```python
from build123d import *

# Parameters (mm, degrees)
BOSS_EXTRUDE1_DEPTH      = 35
SKETCH2_W                = 11
SKETCH2_H                = 21
BOSS_EXTRUDE3_DEPTH      = 150
BOSS_EXTRUDE4_DEPTH      = 35
SKETCH4_W                = 16
SKETCH4_H                = 14
BOSS_EXTRUDE5_DEPTH      = 150
SKETCH5_W                = 14
SKETCH5_H                = 14
BOSS_EXTRUDE6_DEPTH      = 25
SKETCH6_W                = 121
SKETCH6_H                = 207.00216397
BOSS_EXTRUDE7_DEPTH      = 5
SKETCH7_R                = 11
BOSS_EXTRUDE8_DEPTH      = 10
BOSS_EXTRUDE8_DEPTH_BACK = 230
SKETCH8_W                = 46
SKETCH8_H                = 122
CUT_EXTRUDE1_DEPTH       = 5


with BuildPart() as part:
    # Sketch1 → Boss-Extrude1 (new body)
    with BuildSketch(Plane.XY):
        with BuildLine():
            Line((0, 0), (150, 0))
            ThreePointArc((150, 0), (79.056941504, 37.170824513), (0, 50))
            Line((0, 50), (0, 0))
        make_face()
    extrude(amount=BOSS_EXTRUDE1_DEPTH)

    # Sketch2 → Boss-Extrude3 (add)
    with BuildSketch(Plane.XY.offset(35)):
        with Locations((9.5, 24.924601572)):
            Rectangle(SKETCH2_W, SKETCH2_H)
    extrude(amount=BOSS_EXTRUDE3_DEPTH)

    # Sketch3 → Boss-Extrude4 (add)
    with BuildSketch(Plane.XY.offset(185)):
        with BuildLine():
            Line((150, 0), (0, 0))
            Line((0, 0), (0, 50))
            ThreePointArc((0, 50), (79.056941504, 37.170824513), (150, 0))
        make_face()
    extrude(amount=BOSS_EXTRUDE4_DEPTH)

    # Sketch4 → Boss-Extrude5 (add)
    with BuildSketch(Plane(origin=(0, 0, 185), x_dir=(-1, 0, 0), z_dir=(0, 0, -1))):
        with Locations((-102, 13)):
            Rectangle(SKETCH4_W, SKETCH4_H)
    extrude(amount=BOSS_EXTRUDE5_DEPTH)

    # Sketch5 → Boss-Extrude6 (add)
    with BuildSketch(Plane.XZ):
        with Locations((23, 202.48216397)):
            Rectangle(SKETCH5_W, SKETCH5_H)
        with Locations((23, 17.48)):
            Rectangle(SKETCH5_W, SKETCH5_H)
        with Locations((122, 202.48216397)):
            Rectangle(SKETCH5_W, SKETCH5_H)
        with Locations((122, 17.48)):
            Rectangle(SKETCH5_W, SKETCH5_H)
    extrude(amount=BOSS_EXTRUDE6_DEPTH)

    # Sketch6 → Boss-Extrude7 (add)
    with BuildSketch(Plane(origin=(0, -25, 0), x_dir=(-1, 0, 0), z_dir=(0, -1, 0))):
        with Locations((-72.5, -109.981081985)):
            Rectangle(SKETCH6_W, SKETCH6_H)
    extrude(amount=BOSS_EXTRUDE7_DEPTH)

    # Sketch7 → Boss-Extrude8 (add, two sides)
    with BuildSketch(Plane(origin=(0, 0, 0), x_dir=(-1, 0, 0), z_dir=(0, 0, -1))) as boss_extrude8_sk:
        with Locations((-63, 18)):
            Circle(SKETCH7_R)
    extrude(amount=BOSS_EXTRUDE8_DEPTH)
    extrude(boss_extrude8_sk.sketch, amount=-BOSS_EXTRUDE8_DEPTH_BACK)

    # Sketch8 → Cut-Extrude1 (cut)
    with BuildSketch(Plane.XZ.offset(30)):
        with Locations((65, 109.98216397)):
            Rectangle(SKETCH8_W, SKETCH8_H)
    extrude(amount=-CUT_EXTRUDE1_DEPTH, mode=Mode.SUBTRACT)


solid = part.part
```
Geometry check sheet. Reference: the model listing, model coordinates, mm. A direction names the side the tool comes from. Give positions to 0.01 mm unless a question says otherwise; leave off trailing zeros. Order: outer loops, then holes, each group sorted by start corner. A loop starts at its lowest first (then second) coordinate and runs counter-clockwise, first axis right, second up.
1. Section check B-B, the plane z = 121.5. Enter the section's corners in (x, y).
2. Gauge pin test, flat ends, axial feed: pin 1 Ø6.5 at (y, z) = (26.5, 145.5) entering from -X; pin 2 Ø5.5 at (y, z) = (-28, 97.5) entering from -X; pin 3 Ø1.5 at (y, z) = (-26.5, 82.5) entering from +X. Record the tip position at first contact, or that the pin passes through.
3. Release check for a two-part mould opening along X. For faces 1 (the face through (9, 14.425, 109)), 2 (the face through (80.124, 36.812, 17.255)), 3 (the face through (88, -28, 109)), 4 (the face through (12, -27, 111)) record: pulls with the +X half, pulls with the -X half, needs draft (parallel to the pull), parting line crosses it, or undercut.
4. Section check D-D, the plane x = 63. Enter the section's corners in (y, z).
5. Access from +Z, -Z, +X, -X, +Y, -Y to the whole of each face (thin tool, end or side, straight path). Record for faces 5 (the face through (102, 20, 111)), 6 (the face through (15, 25, 109)), 7 (the face through (115, -12, 17)), 8 (the face through (65, -28, 48.982)), 9 (the face through (71.73, 11.31, -4.93)).
6. Section check A-A, the plane z = 31.5. Enter the section's corners in (x, y), and give its area (3 significant figures).
7. Thickness scan on L1, parallel to Y at x = 104.5, z = 98; L2, parallel to Z at x = 58.5, y = 6.5; L3, parallel to Z at x = 120, y = -24.5. Record the ranges inside material, lowest first.
8. Section check C-C, the plane x = 97.5. Enter the section's corners in (y, z), and give its area (3 significant figures).
Values follow:
1. outline: (4, 14.42) - (15, 14.42) - (15, 35.42) - (4, 35.42) - close; (12, -30) - (42, -30) - (42, -25) - (12, -25) - close; circle Ø22 at (63, 18); (88, -30) - (133, -30) - (133, -25) - (88, -25) - close; (94, 6) - (110, 6) - (110, 20) - (94, 20) - close
2. pin 1: stops at x = 4
2. pin 2: stops at x = 12
2. pin 3: stops at x = 133
3. face 1: needs draft
3. face 2: pulls with the +X half
3. face 3: undercut
3. face 4: pulls with the -X half
4. outline: (-30, 6.48) - (-25, 6.48) - (-25, 48.98) - (-30, 48.98) - close; (-30, 170.98) - (-25, 170.98) - (-25, 213.48) - (-30, 213.48) - close; (0, 0) - (7, 0) - (7, -10) - (29, -10) - (29, 0) - (41.93, 0) - (41.93, 35) - (29, 35) - (29, 185) - (41.93, 185) - (41.93, 220) - (29, 220) - (29, 230) - (7, 230) - (7, 220) - (0, 220) - (0, 185) - (7, 185) - (7, 35) - (0, 35) - close
5. face 5: +X, +Y
5. face 6: +Y
5. face 7: +Z, -Z
5. face 8: -Y
5. face 9: -Z
6. outline: (0, 0) - (150, 0) arc R250 ccw to (0, 50) - close; (12, -30) - (133, -30) - (133, -25) - (12, -25) - close
6. area: 5,710 mm2
7. L1: y = -30 to -25, 6 to 20
7. L2: z = 0 to 35, 185 to 220
7. L3: z = 10.48 to 24.48, 195.48 to 209.48
8. outline: (-30, 6.48) - (-25, 6.48) - (-25, 213.48) - (-30, 213.48) - close; (0, 0) - (30.2, 0) - (30.2, 35) - (20, 35) - (20, 185) - (30.2, 185) - (30.2, 220) - (0, 220) - (0, 185) - (6, 185) - (6, 35) - (0, 35) - close
8. area: 5,250 mm2
